The model under review builds one solid part; all positions refer to its coordinate system, in mm. Face numbers are marked on the shaded views. A direction names the side the tool comes from. Coordinates: 2 decimals unless noted, no trailing zeros. Loops run counter-clockwise (first coordinate to the right, second up) from the corner with the lowest first, then second, coordinate; pieces in that order, holes last. Notation, with made-up numbers: (4, 73) - (62, 73) arc R31 ccw to (62, 104) - close; hole circle Ø3 at (66, 55.5). An arc over 180 degrees is marked (long way). One line per item, written item: value. Start each with the question number.
1. We need section A-A, the plane z = -11.5. Give the boundary of the cut face in (x, y), then the cut area to 3 significant figures.
2. Mouldability with a two-part tool opening along Y and no side actions: class the marked faces 4, 5 and 6 as +Y half, -Y half, draft (parallel to the pull), parting line (faces both ways), or undercut.
3. Insertion check: P1, Ø6, axis at x = -3, y = -27.5, coming from the -Z side. The pin has a flat end and moves straight along its axis. Give the tip position at first contact, or say it passes through.
4. We need section B-B, the plane y = -30. Give the boundary of the cut face in (x, z), then the cut area to 3 significant figures.
5. We need section D-D, the plane x = -47.5. Give the boundary of the cut face in (y, z), then the cut area to 3 significant figures.
6. For the marked faces 1, 2 and 3, list the 3-axis set-ups (+Z, -Z, +X, -X, +Y, -Y) from which the entire face can be reached by the end or side of a thin tool; tool diameter is ignored.
7. We need section C-C, the plane z = 15. Give the boundary of the cut face in (x, y), then the cut area to 3 significant figures.
8. To check wall thickness, follow line 1 (X direction, y = -30, z = -6); line 2 (Z direction, x = -18.5, y = -4); line 3 (X direction, y = -39, z = 13.5). State the ranges of each line that lie inside material, in increasing order.
from build123d import *

# Parameters (mm, degrees)
F1_DEPTH = 60
F3_DEPTH = 15


with BuildPart() as f1:
    # F0 (on Front) → F1 (new body)
    with BuildSketch(Plane.XZ):
        Polygon((60, 17), (-60, 17), (-60, -17), (-20, -17), (-20, -5), (20, -5), (20, -17), (60, -17), align=None)
    extrude(amount=F1_DEPTH)

    # F2 (on face) → F3 (cut)
    with BuildSketch(Plane.XY.offset(17)):
        with BuildLine():
            ThreePointArc((-60, -45), (-45, -30), (-60, -15))
            Line((-60, -15), (-60, -45))
        make_face()
        with BuildLine():
            Line((60, -45), (60, -15))
            ThreePointArc((60, -15), (45, -30), (60, -45))
        make_face()
    extrude(amount=-F3_DEPTH, mode=Mode.SUBTRACT)


solid = f1.part
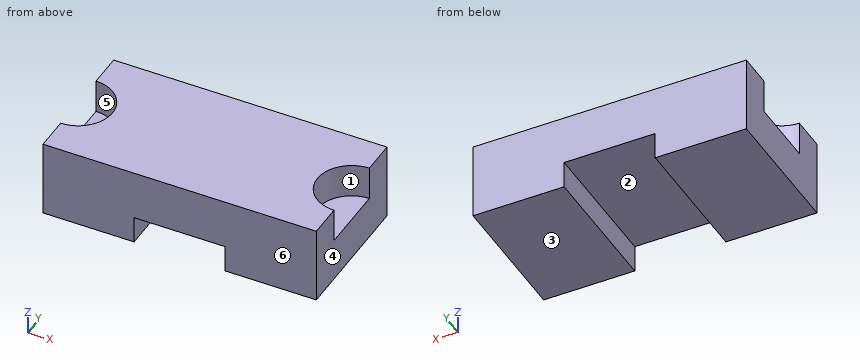
Findings below:
1. outline: (-60, -60) - (-20, -60) - (-20, 0) - (-60, 0) - close; (20, -60) - (60, -60) - (60, 0) - (20, 0) - close
1. area: 4,800 mm2
2. face 4: draft
2. face 5: undercut
2. face 6: -Y half
3. P1: z = -5
4. outline: (-60, -17) - (-20, -17) - (-20, -5) - (20, -5) - (20, -17) - (60, -17) - (60, 2) - (45, 2) - (45, 17) - (-45, 17) - (-45, 2) - (-60, 2) - close
4. area: 3,150 mm2
5. outline: (-60, -17) - (0, -17) - (0, 17) - (-21.71, 17) - (-21.71, 2) - (-38.29, 2) - (-38.29, 17) - (-60, 17) - close
5. area: 1,790 mm2
6. face 1: +Z, +X
6. face 2: -Z, +Y, -Y
6. face 3: -Z, +X, -X, +Y, -Y
7. outline: (-60, -60) - (60, -60) - (60, -45) arc R15 cw to (60, -15) - (60, 0) - (-60, 0) - (-60, -15) arc R15 cw to (-60, -45) - close
7. area: 6,490 mm2
8. line 1: -60 to -20, 20 to 60
8. line 2: -5 to 17
8. line 3: -48 to 48
